Here's the drawing with two shaded views (mm, measured from the low corner). I have some questions. Round coordinates to 2 decimals unless told otherwise and drop trailing zeros. Loops run counter-clockwise (first coordinate to the right, second up) from the corner with the lowest first, then second, coordinate; pieces in that order, holes last. Notation, with made-up numbers: (18.25, 11) -> (45.25, 11) arc R26 cw to (45.25, 34) -> close; hole circle Ø4 at (21.25, 24.5). An arc over 180 degrees is marked (long way). One line per item, written item: value. Start each with the question number.
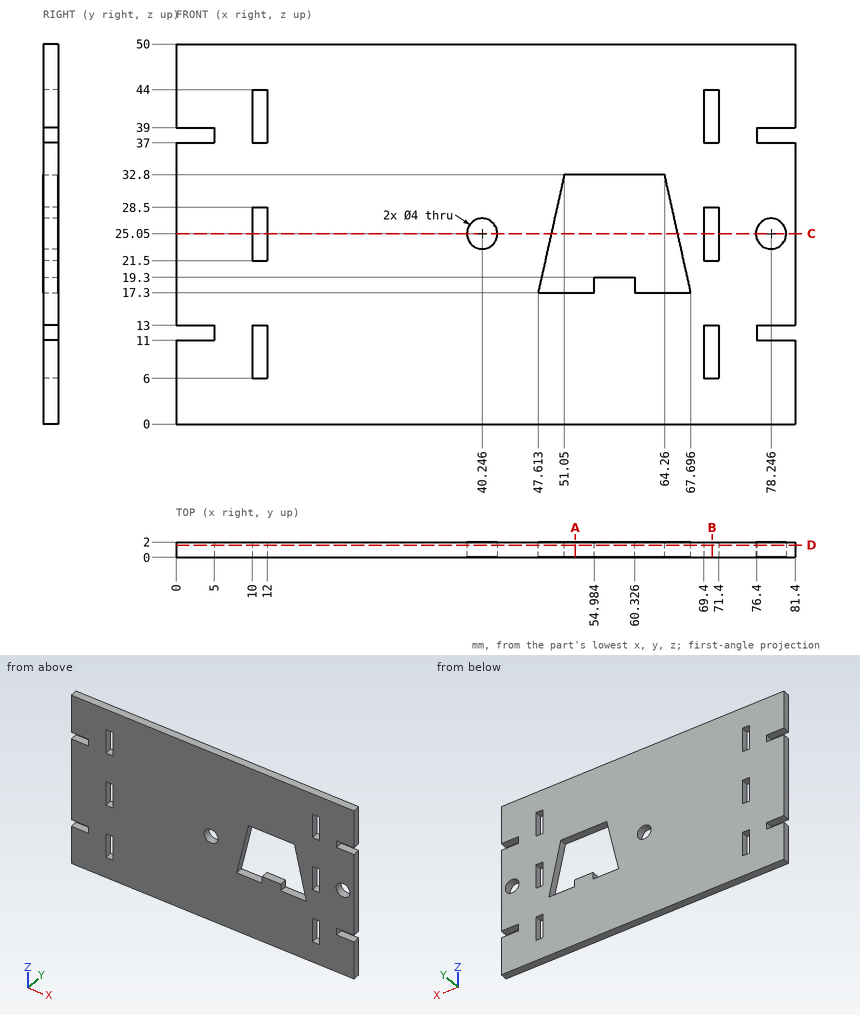
Q1. I want a section at A-A on x = 52.5. Please give me the cut outline in (y, z).
Q2. I want a section at B-B on x = 70.5. Please give me the cut outline in (y, z).
Q3. I want a section at C-C on z = 25.05. Please give me the cut outline in (x, y).
Q4. I want a section at D-D on y = 1.6. State how many separate pieces and enclosed holes the cut face has, plus the area to 3 significant figures.
Q5. If I drill on line 1 along X through (y, z) = (0.4, 38.5); line 2 along Z through (x, y) = (71, 0.4); line 3 along X through (y, z) = (0.8, 25.05), over which ranges is the centre line in solid material (lowest first)?
Answers below:
1. outline: (0, 0) -> (2, 0) -> (2, 17.3) -> (0, 17.3) -> close; (0, 32.8) -> (2, 32.8) -> (2, 50) -> (0, 50) -> close
2. outline: (0, 0) -> (2, 0) -> (2, 6) -> (0, 6) -> close; (0, 13) -> (2, 13) -> (2, 21.5) -> (0, 21.5) -> close; (0, 28.5) -> (2, 28.5) -> (2, 37) -> (0, 37) -> close; (0, 44) -> (2, 44) -> (2, 50) -> (0, 50) -> close
3. outline: (0, 0) -> (10, 0) -> (10, 2) -> (0, 2) -> close; (12, 0) -> (38.25, 0) -> (38.25, 2) -> (12, 2) -> close; (42.25, 0) -> (49.33, 0) -> (49.33, 2) -> (42.25, 2) -> close; (65.98, 0) -> (69.4, 0) -> (69.4, 2) -> (65.98, 2) -> close; (71.4, 0) -> (76.25, 0) -> (76.25, 2) -> (71.4, 2) -> close; (80.25, 0) -> (81.4, 0) -> (81.4, 2) -> (80.25, 2) -> close
4. separate pieces: 1
4. enclosed holes: 9
4. area: 3,670 mm^2
5. line 1: x = 5 to 10, 12 to 69.4, 71.4 to 76.4
5. line 2: z = 0 to 6, 13 to 21.5, 28.5 to 37, 44 to 50
5. line 3: x = 0 to 10, 12 to 38.25, 42.25 to 49.33, 65.98 to 69.4, 71.4 to 76.25, 80.25 to 81.4
